Check sheet for the drawn part. Datum: minimum x, y, z corner. Units: mm. Give positions to 0.01 mm unless a question says otherwise; leave off trailing zeros. Order: outer loops, then holes, each group sorted by start corner. A loop starts at its lowest first (then second) coordinate and runs counter-clockwise, first axis right, second up.
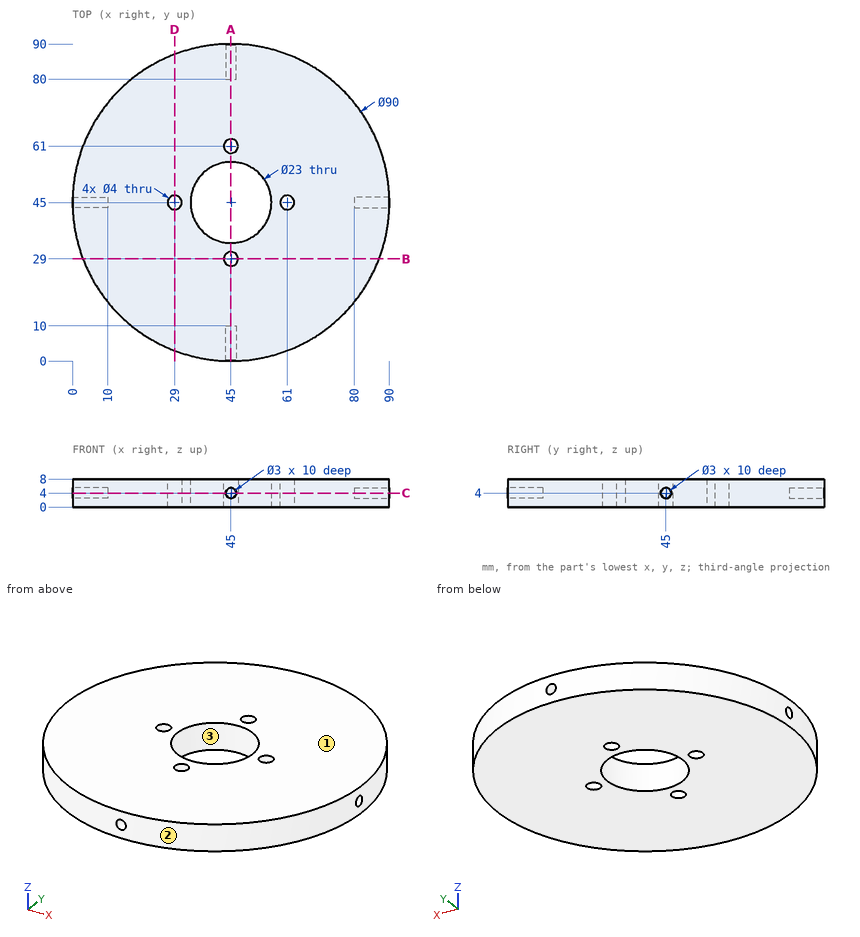
Item 1: Draft check along X on the marked faces 1, 2 and 3. Enter one of: released by +X, released by -X, zero draft, split by the parting line, or undercut.
Reported:
face 1: zero draft
face 2: split by the parting line
face 3: undercut
Item 2: Gauge pin test, flat ends, axial feed: pin 1 (1.5 mm diameter, centred on x = 58, z = 2, fed in from -Y); pin 2 (2 mm diameter, centred on y = 13.5, z = 3.5, fed in from -X); pin 3 (0.9 mm diameter, centred on x = 45.5, z = 4, fed in from -Y). Record the tip position at first contact, or that the pin passes through.
Reported:
pin 1: stops at y = 1.7
pin 2: stops at x = 11.91
pin 3: stops at y = 10
Item 3: Sectioned sample at C-C (z = 4). Enter the section's corners in (x, y) (3 decimals).
Reported:
outline: (0.025, 43.5) arc R45 ccw to (43.5, 0.025) - (43.5, 10) - (46.5, 10) - (46.5, 0.025) arc R45 ccw to (89.975, 43.5) - (80, 43.5) - (80, 46.5) - (89.975, 46.5) arc R45 ccw to (46.5, 89.975) - (46.5, 80) - (43.5, 80) - (43.5, 89.975) arc R45 ccw to (0.025, 46.5) - (10, 46.5) - (10, 43.5) - close; hole circle Ø4 at (29, 45); hole circle Ø23 at (45, 45); hole circle Ø4 at (45, 29); hole circle Ø4 at (45, 61); hole circle Ø4 at (61, 45)
Item 4: Scan lines: L1, parallel to Y at x = 45, z = 3.75; L2, parallel to X at y = 41.5, z = 4.5; L3, parallel to Y at x = 29, z = 3.5. Record each from-to range of solid material in increasing order.
Reported:
L1: y = 10 to 27, 31 to 33.5, 56.5 to 59, 63 to 80
L2: x = 0.14 to 34.05, 55.95 to 89.86
L3: y = 2.94 to 43, 47 to 87.06
Item 5: Sectioned sample at A-A (x = 45). Enter the section's corners in (y, z).
Reported:
outline: (0, 0) - (27, 0) - (27, 8) - (0, 8) - (0, 5.5) - (10, 5.5) - (10, 2.5) - (0, 2.5) - close; (31, 0) - (33.5, 0) - (33.5, 8) - (31, 8) - close; (56.5, 0) - (59, 0) - (59, 8) - (56.5, 8) - close; (63, 0) - (90, 0) - (90, 2.5) - (80, 2.5) - (80, 5.5) - (90, 5.5) - (90, 8) - (63, 8) - close
Item 6: Sectioned sample at B-B (y = 29). Enter the section's corners in (x, z), and give its area (3 significant figures).
Reported:
outline: (2.94, 0) - (43, 0) - (43, 8) - (2.94, 8) - close; (47, 0) - (87.06, 0) - (87.06, 8) - (47, 8) - close
area: 641 mm2
